Source: CAD feature listing. Evaluate the final solid. Frame: model axes, mm. Face numbers are marked on the shaded views. Round coordinates to 2 decimals unless told otherwise and drop trailing zeros. Write each loop counter-clockwise with the first axis right and the second up, starting at its lowest first coordinate (ties: lowest second). Pieces come first, ordered by that corner, then holes. Notation, with made-up numbers: M -10.75,55 L 36.25,55 A24 cw 36.25,72 Z; hole C -2,-13 d10. An arc over 180 degrees is marked long. Put each result on its own line as item: value. Start each with the question number.
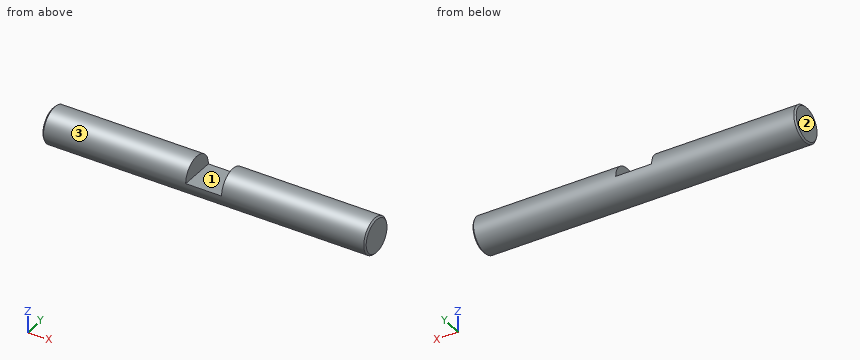
Solid Edge part; units mm, degrees
sketch "Sketch1" plane through (0, 0, 0) normal (1, 0, 0) x (0, 1, 0)
  circle A0 centre (0, 0) radius 1.5
extrude "Protrusion1" add sketch "Sketch1" along normal mid plane 27
sketch "Sketch2" plane through (0, 0, 0) normal (0, -1, 0) x (1, 0, 0)
  line L0 (-1.5, 1.5) -> (-1.5, 0)
  line L1 (-1.5, 0) -> (1.5, 0)
  line L2 (1.5, 0) -> (1.5, 1.5)
  dimension "D1" = 1.5
extrude "Extrusionsausschnitt_1" cut sketch "Sketch2" along normal mid plane 28 material side at (-1.45, 0, 0.75)
chamfer "Fase_1" distance 0.125 angle 45 2 edges at (13.5, -1.5, 0) (-13.5, -1.5, 0)
(1) Section query A-A (y = 0). Return loops of the section in (x, z) (3 decimals).
(2) Ray query, line 1 along X through (y, z) = (-0.15, 0.55); line 2 along Z through (x, y) = (0.5, -0.6); line 3 along Z through (x, y) = (6.5, -1). Return the intervals inside material, ascending.
(3) Pull-direction query (X, two-part tool) for the marked faces 1, 2 and 3; classes: +X half, -X half, draft (parallel to the pull), parting line (faces both ways), or undercut.
(4) Section query B-B (x = 2). Return loops of the section in (y, z), and give its area (3 significant figures).
(5) Contact query for a flat-ended pin moving along its axis: P1, Ø0.9, axis at x = 0, y = 0.5, coming from the +Z side. Output: stop coordinate, or through.
Entries:
1. outline: M -13.5,-1.375 L -13.375,-1.5 L 13.375,-1.5 L 13.5,-1.375 L 13.5,1.375 L 13.375,1.5 L 1.5,1.5 L 1.5,0 L -1.5,0 L -1.5,1.5 L -13.375,1.5 L -13.5,1.375 Z
2. line 1: -13.5 to -1.5, 1.5 to 13.5
2. line 2: -1.37 to 0
2. line 3: -1.12 to 1.12
3. face 1: undercut
3. face 2: -X half
3. face 3: draft
4. outline: C 0,0 d3
4. area: 7.07 mm2
5. P1: z = 0
